Could you check a few things on this model? Use its own coordinates, in mm. Face numbers are marked on the shaded views. A direction names the side the tool comes from. Give positions to 0.01 mm unless a question says otherwise; leave off trailing zeros. Loops run counter-clockwise (first coordinate to the right, second up) from the corner with the lowest first, then second, coordinate; pieces in that order, holes last. Notation, with made-up numbers: (-17.5, 87) - (-10.5, 87) arc R27 ccw to (-10.5, 106) - close; hole circle Ø5 at (-30, 22). An arc over 180 degrees is marked (long way). One line per item, written item: value. Start each with the question number.
Q1. I want a section at C-C (x = 0). Please give me the cut outline in (y, z) (3 decimals), then the cut area to 3 significant figures.
Q2. For the marked faces 1 and 2, which set-ups out of +Z, -Z, +X, -X, +Y, -Y let a thin tool reach every point of the face, with its end or its side?
Q3. I want a section at D-D (z = -2). Please give me the cut outline in (x, y), then the cut area to 3 significant figures.
Q4. I'm going to push flat-ended pins straight in: P1, Ø1.5, axis at x = 0.5, y = 5, coming from the +Z side (3 decimals); P2, Ø1, axis at y = 8, z = -10, coming from the -X side; P3, Ø1, axis at x = 22.5, y = 3, coming from the -Z side. Where does each tip first touch, or does it pass through?
Q5. I want a section at A-A (z = -4.75). Please give me the cut outline in (x, y), then the cut area to 3 significant figures.
Q6. If we mould it in two halves opening along X, with no side actions, what happens to the marked faces 3, 4, 5 and 6? For each: released by +X, released by -X, zero draft, split by the parting line, or undercut.
Q7. If I drill on line 1 (X direction, y = 8.5, z = 0.25); line 2 (Y direction, x = 3, z = 5.25); line 3 (X direction, y = 9, z = -1.75), over which ranges is the centre line in solid material (lowest first)? Write a range as from..to.
Q8. I want a section at B-B (y = 8.25). Please give me the cut outline in (x, z) (3 decimals), then the cut area to 3 significant figures.
```python
from build123d import *

# Parameters (mm, degrees)
F0_R     = 3.175
F1_DEPTH = 10.16
F2_W     = 5.08
F2_H     = 13.335
F3_DEPTH = 12.7
F4_R     = 1.5748


with BuildPart() as f1:
    # F0 (on Front) → F1 (new body)
    with BuildSketch(Plane.XZ):
        with BuildLine():
            ThreePointArc((6.132791, -8.89), (4.348923, -6.627547), (5.060618, -3.835707))
            ThreePointArc((5.060618, -3.835707), (2.023311, 6.019029), (-6.35, 0))
            ThreePointArc((-6.35, 0), (-2.471626, -8.672607), (6.132791, -12.7))
            ThreePointArc((6.132791, -12.7), (23.253233, -14.268605), (40.373676, -12.7))
            Line((40.373676, -12.7), (40.373676, -8.89))
            ThreePointArc((40.373676, -8.89), (23.253233, -10.614816), (6.132791, -8.89))
        make_face()
        with Locations((-1.143, 0)):
            Circle(F0_R, mode=Mode.SUBTRACT)
    extrude(amount=-F1_DEPTH)

    # F2 (on Right) → F3 (cut, symmetric)
    with BuildSketch(Plane.YZ):
        with Locations((5.08, 0.9525)):
            Rectangle(F2_W, F2_H)
    extrude(amount=F3_DEPTH, both=True, mode=Mode.SUBTRACT)

    # F4
    f4_edges = [f1.edges().sort_by_distance(p)[0] for p in [
        (40.373676, 5.08, -8.89),
        (40.373676, 5.08, -12.7),
    ]]
    fillet(f4_edges, radius=F4_R)


solid = f1.part
```
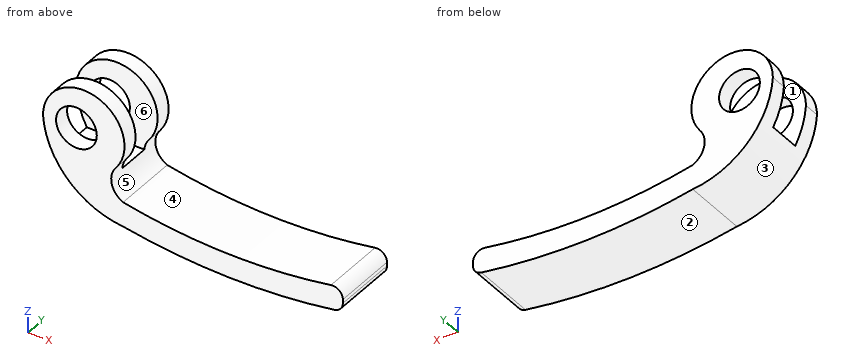
Worked answers:
1. outline: (0, -10.66) - (10.16, -10.66) - (10.16, -2.962) - (7.62, -2.962) - (7.62, -5.715) - (2.54, -5.715) - (2.54, -2.962) - (0, -2.962) - close; (0, 2.962) - (2.54, 2.962) - (2.54, 6.35) - (0, 6.35) - close; (7.62, 2.962) - (10.16, 2.962) - (10.16, 6.35) - (7.62, 6.35) - close
1. area: 81.4 mm²
2. face 1: +Z, +X, -X
2. face 2: -Z, +Y, -Y
3. outline: (-6.07, 0) - (-3.61, 0) - (-3.61, 2.54) - (-6.07, 2.54) - close; (-6.07, 7.62) - (-3.61, 7.62) - (-3.61, 10.16) - (-6.07, 10.16) - close; (1.32, 0) - (6.03, 0) - (6.03, 2.54) - (1.32, 2.54) - close; (1.32, 7.62) - (6.03, 7.62) - (6.03, 10.16) - (1.32, 10.16) - close
3. area: 36.4 mm²
4. P1: stops at z = -5.715
4. P2: stops at x = -1.58
4. P3: stops at z = -14.27
5. outline: (-5.16, 0) - (4.51, 0) - (4.51, 2.54) - (-5.16, 2.54) - close; (-5.16, 7.62) - (4.51, 7.62) - (4.51, 10.16) - (-5.16, 10.16) - close
5. area: 49.1 mm²
6. face 3: released by -X
6. face 4: undercut
6. face 5: released by +X
6. face 6: zero draft
7. line 1: x = -6.35..-4.31, 2.02..6.35
7. line 2: y = 0..2.54, 7.62..10.16
7. line 3: x = -6.12..-3.79, 1.51..6.1
8. outline: (-6.35, 0) arc R13.62 ccw to (6.133, -12.7) arc R94.214 ccw to (39.063, -12.933) arc R1.575 ccw to (40.374, -11.38) - (40.374, -10.796) arc R1.575 ccw to (38.519, -9.246) arc R85.831 cw to (6.133, -8.89) arc R3.254 cw to (5.061, -3.836) arc R6.35 ccw (long way) to start; hole circle Ø6.35 at (-1.143, 0)
8. area: 269 mm²
